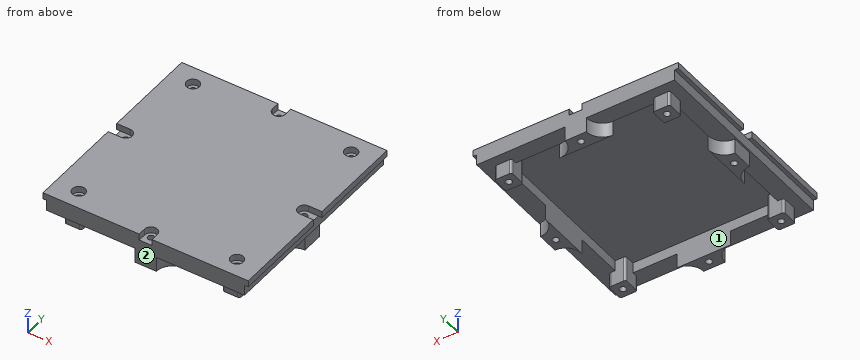
from build123d import *
from build123d.topology import SkipClean

# Parameters (mm, degrees)
SKETCH3_W           = 96
SKETCH3_H           = 3
BOSS_EXTRUDE1_DEPTH = 96
SKETCH4_R           = 1.5
BOSS_EXTRUDE2_DEPTH = 12
SKETCH5_R           = 1.5
BOSS_EXTRUDE3_DEPTH = 12
BOSS_EXTRUDE4_DEPTH = 5
SKETCH10_R          = 1.5
CUT_EXTRUDE1_DEPTH  = 70.519781358
SKETCH11_R          = 3
CUT_EXTRUDE2_DEPTH  = 3
CUT_EXTRUDE3_DEPTH  = 3


with BuildPart() as part:
    # Sketch3 → Boss-Extrude1 (new body)
    with BuildSketch(Plane(origin=(0, 48, 0), x_dir=(1, 0, 0), z_dir=(0, 1, 0))):
        with Locations((0, -1.5)):
            Rectangle(SKETCH3_W, SKETCH3_H)
    extrude(amount=-BOSS_EXTRUDE1_DEPTH)

    # Sketch4 → Boss-Extrude2 (add)
    # profile 1 of 4: a face of its own
    with BuildSketch(Plane(origin=(0, 0, 0), x_dir=(-1, 0, 0), z_dir=(0, 0, -1))):
        with BuildLine():
            Line((38, -12.5), (38, 12.5))
            ThreePointArc((38, 12.5), (40.196699141, 7.196699141), (45.5, 5))
            Line((45.5, 5), (45.5, -5))
            ThreePointArc((45.5, -5), (40.196699141, -7.196699141), (38, -12.5))
        make_face()
        with Locations(Location((41.75, 0, 0), (0, 0, 180))):
            Circle(SKETCH4_R, mode=Mode.SUBTRACT)
    # profile 2 of 4: a face of its own
    with BuildSketch(Plane(origin=(0, 0, 0), x_dir=(-1, 0, 0), z_dir=(0, 0, -1))):
        with BuildLine():
            Line((12.5, 40.5), (-12.5, 40.5))
            ThreePointArc((-12.5, 40.5), (-7.196699141, 42.696699141), (-5, 48))
            Line((-5, 48), (5, 48))
            ThreePointArc((5, 48), (7.196699141, 42.696699141), (12.5, 40.5))
        make_face()
        with Locations(Location((0, 44.25, 0), (0, 0, 180))):
            Circle(SKETCH4_R, mode=Mode.SUBTRACT)
    # profile 3 of 4: a face of its own
    with BuildSketch(Plane(origin=(0, 0, 0), x_dir=(-1, 0, 0), z_dir=(0, 0, -1))):
        with BuildLine():
            Line((-5, -48), (5, -48))
            ThreePointArc((5, -48), (7.196699141, -42.696699141), (12.5, -40.5))
            Line((12.5, -40.5), (-12.5, -40.5))
            ThreePointArc((-12.5, -40.5), (-7.196699141, -42.696699141), (-5, -48))
        make_face()
        with Locations(Location((0, -44.25, 0), (0, 0, 180))):
            Circle(SKETCH4_R, mode=Mode.SUBTRACT)
    # profile 4 of 4: a face of its own
    with BuildSketch(Plane(origin=(0, 0, 0), x_dir=(-1, 0, 0), z_dir=(0, 0, -1))):
        with BuildLine():
            Line((-45.5, 5), (-45.5, -5))
            ThreePointArc((-45.5, -5), (-40.196699141, -7.196699141), (-38, -12.5))
            Line((-38, -12.5), (-38, 12.5))
            ThreePointArc((-38, 12.5), (-40.196699141, 7.196699141), (-45.5, 5))
        make_face()
        with Locations(Location((-41.75, 0, 0), (0, 0, 180))):
            Circle(SKETCH4_R, mode=Mode.SUBTRACT)
    extrude(amount=BOSS_EXTRUDE2_DEPTH)

    # Sketch5 → Boss-Extrude3 (add)
    # profile 1 of 4: a face of its own
    with BuildSketch(Plane(origin=(0, 0, 0), x_dir=(-1, 0, 0), z_dir=(0, 0, -1))):
        with BuildLine():
            Line((-40, 35.5), (-34, 35.5))
            ThreePointArc((-34, 35.5), (-33.292893219, 35.792893219), (-33, 36.5))
            Line((-33, 36.5), (-33, 42.5))
            ThreePointArc((-33, 42.5), (-33.292893219, 43.207106781), (-34, 43.5))
            Line((-34, 43.5), (-40, 43.5))
            ThreePointArc((-40, 43.5), (-40.707106781, 43.207106781), (-41, 42.5))
            Line((-41, 42.5), (-41, 36.5))
            ThreePointArc((-41, 36.5), (-40.707106781, 35.792893219), (-40, 35.5))
        make_face()
        with Locations(Location((-37, 39.5, 0), (0, 0, 90))):
            Circle(SKETCH5_R, mode=Mode.SUBTRACT)
    # profile 2 of 4: a face of its own
    with BuildSketch(Plane(origin=(0, 0, 0), x_dir=(-1, 0, 0), z_dir=(0, 0, -1))):
        with BuildLine():
            Line((33, 36.5), (33, 42.5))
            ThreePointArc((33, 42.5), (33.292893219, 43.207106781), (34, 43.5))
            Line((34, 43.5), (40, 43.5))
            ThreePointArc((40, 43.5), (40.707106781, 43.207106781), (41, 42.5))
            Line((41, 42.5), (41, 36.5))
            ThreePointArc((41, 36.5), (40.707106781, 35.792893219), (40, 35.5))
            Line((40, 35.5), (34, 35.5))
            ThreePointArc((34, 35.5), (33.292893219, 35.792893219), (33, 36.5))
        make_face()
        with Locations(Location((37, 39.5, 0), (0, 0, 90))):
            Circle(SKETCH5_R, mode=Mode.SUBTRACT)
    # profile 3 of 4: a face of its own
    with BuildSketch(Plane(origin=(0, 0, 0), x_dir=(-1, 0, 0), z_dir=(0, 0, -1))):
        with BuildLine():
            Line((-33, -36.5), (-33, -42.5))
            ThreePointArc((-33, -42.5), (-33.292893219, -43.207106781), (-34, -43.5))
            Line((-34, -43.5), (-40, -43.5))
            ThreePointArc((-40, -43.5), (-40.707106781, -43.207106781), (-41, -42.5))
            Line((-41, -42.5), (-41, -36.5))
            ThreePointArc((-41, -36.5), (-40.707106781, -35.792893219), (-40, -35.5))
            Line((-40, -35.5), (-34, -35.5))
            ThreePointArc((-34, -35.5), (-33.292893219, -35.792893219), (-33, -36.5))
        make_face()
        with Locations(Location((-37, -39.5, 0), (0, 0, 90))):
            Circle(SKETCH5_R, mode=Mode.SUBTRACT)
    # profile 4 of 4: a face of its own
    with BuildSketch(Plane(origin=(0, 0, 0), x_dir=(-1, 0, 0), z_dir=(0, 0, -1))):
        with BuildLine():
            Line((40, -35.5), (34, -35.5))
            ThreePointArc((34, -35.5), (33.292893219, -35.792893219), (33, -36.5))
            Line((33, -36.5), (33, -42.5))
            ThreePointArc((33, -42.5), (33.292893219, -43.207106781), (34, -43.5))
            Line((34, -43.5), (40, -43.5))
            ThreePointArc((40, -43.5), (40.707106781, -43.207106781), (41, -42.5))
            Line((41, -42.5), (41, -36.5))
            ThreePointArc((41, -36.5), (40.707106781, -35.792893219), (40, -35.5))
        make_face()
        with Locations(Location((37, -39.5, 0), (0, 0, 90))):
            Circle(SKETCH5_R, mode=Mode.SUBTRACT)
    extrude(amount=BOSS_EXTRUDE3_DEPTH)

    # Sketch8 → Boss-Extrude4 (add)
    with BuildSketch(Plane(origin=(0, 0, 0), x_dir=(-1, 0, 0), z_dir=(0, 0, -1))):
        with BuildLine():
            Line((-38, 40.5), (-12.5, 40.5))
            ThreePointArc((-12.5, 40.5), (-7.196699141, 42.696699141), (-5, 48))
            Line((-5, 48), (-46.25, 48))
            Line((-46.25, 48), (-46.25, -48))
            Line((-46.25, -48), (-5, -48))
            ThreePointArc((-5, -48), (-7.196699141, -42.696699141), (-12.5, -40.5))
            Line((-12.5, -40.5), (-38, -40.5))
            Line((-38, -40.5), (-38, 40.5))
        make_face()
        with BuildLine():
            Line((12.5, 40.5), (38, 40.5))
            Line((38, 40.5), (38, -40.5))
            Line((38, -40.5), (12.5, -40.5))
            ThreePointArc((12.5, -40.5), (7.196699141, -42.696699141), (5, -48))
            Line((5, -48), (46.25, -48))
            Line((46.25, -48), (46.25, 48))
            Line((46.25, 48), (5, 48))
            ThreePointArc((5, 48), (7.196699141, 42.696699141), (12.5, 40.5))
        make_face()
    extrude(amount=BOSS_EXTRUDE4_DEPTH)

    # Sketch10 → Cut-Extrude1 (cut, through all)
    with BuildSketch(Plane.XY.offset(3)):
        with Locations((37, -39.5)):
            Circle(SKETCH10_R)
        with Locations((0, -44.25)):
            Circle(SKETCH10_R)
        with Locations((-37, -39.5)):
            Circle(SKETCH10_R)
        with Locations((-41.75, 0)):
            Circle(SKETCH10_R)
        with Locations((-37, 39.5)):
            Circle(SKETCH10_R)
        with Locations((0, 44.25)):
            Circle(SKETCH10_R)
        with Locations((37, 39.5)):
            Circle(SKETCH10_R)
        with Locations((41.75, 0)):
            Circle(SKETCH10_R)
    extrude(amount=-CUT_EXTRUDE1_DEPTH, mode=Mode.SUBTRACT)

    # Sketch11 → Cut-Extrude2 (cut)
    with SkipClean():  # the faces are left unmerged after this step: merging them gives an invalid solid
        with BuildSketch(Plane.XY.offset(3)):
            with Locations((0, -44.25)):
                Circle(SKETCH11_R)
            with Locations((-37, -39.5)):
                Circle(SKETCH11_R)
            with Locations((-41.75, 0)):
                Circle(SKETCH11_R)
            with Locations((-37, 39.5)):
                Circle(SKETCH11_R)
            with Locations((0, 44.25)):
                Circle(SKETCH11_R)
            with Locations(Location((37, -39.5, 0), (0, 0, 180))):
                Circle(SKETCH11_R)
            with Locations(Location((41.75, 0, 0), (0, 0, 180))):
                Circle(SKETCH11_R)
            with Locations(Location((37, 39.5, 0), (0, 0, 180))):
                Circle(SKETCH11_R)
        extrude(amount=-CUT_EXTRUDE2_DEPTH, mode=Mode.SUBTRACT)

    # Sketch12 → Cut-Extrude3 (cut)
    with BuildSketch(Plane.XY.offset(3)):
        with BuildLine():
            Line((3, -44.25), (3, -51.044271795))
            Line((3, -51.044271795), (-3, -51.044271795))
            Line((-3, -51.044271795), (-3, -44.24999935))
            ThreePointArc((-3, -44.24999935), (-3.25e-07, -47.25), (3, -44.25))
        make_face()
        with BuildLine():
            Line((3, 44.25), (3, 51.044271795))
            Line((3, 51.044271795), (-3, 51.044271795))
            Line((-3, 51.044271795), (-3, 44.24999935))
            ThreePointArc((-3, 44.24999935), (-3.25e-07, 47.25), (3, 44.25))
        make_face()
        with BuildLine():
            Line((41.75, -3), (50.168428877, -3))
            Line((50.168428877, -3), (50.168428877, 3))
            Line((50.168428877, 3), (41.75, 3))
            ThreePointArc((41.75, 3), (44.75, 0), (41.75, -3))
        make_face()
        with BuildLine():
            Line((-50.168428877, -3), (-50.168428877, 3))
            Line((-50.168428877, 3), (-41.75, 3))
            ThreePointArc((-41.75, 3), (-44.75, 0), (-41.75, -3))
            Line((-41.75, -3), (-50.168428877, -3))
        make_face()
    extrude(amount=-CUT_EXTRUDE3_DEPTH, mode=Mode.SUBTRACT)


solid = part.part
Geometry check sheet. Reference: the model listing, model coordinates, mm. Face numbers are marked on the shaded views. A direction names the side the tool comes from. Give positions to 0.01 mm unless a question says otherwise; leave off trailing zeros. Loops run counter-clockwise (first coordinate to the right, second up) from the corner with the lowest first, then second, coordinate; pieces in that order, holes last. Notation, with made-up numbers: M 47,83 L 103,83 A31 cw 103,117 Z; hole C 16,-7.5 d11. An arc over 180 degrees is marked long. Answer as a JSON object with one key per item and string values. Group by question number.
Item 1: Sectioned sample at C-C on y = 27. Record the boundary of the cut face in (x, z).
Item 2: Material ranges on L1, parallel to Y at x = 37, z = -2.25; L2, parallel to Y at x = -37, z = 0.5; L3, parallel to X at y = -37.5, z = -8, recorded low to high.
Item 3: Sectioned sample at A-A on z = -3.5. Give the number of separate pieces and of enclosed holes in the cut face, plus the area to 3 significant figures.
Item 4: Access from +Z, -Z, +X, -X, +Y, -Y to the whole of each face (thin tool, end or side, straight path). Record for the marked faces 1 and 2.
Item 5: Gauge pin test, flat ends, axial feed: pin 1 (6 mm diameter, centred on x = 28, y = 8, fed in from -Z); pin 2 (6.5 mm diameter, centred on x = 37.5, y = 39, fed in from +Z); pin 3 (2.5 mm diameter, centred on x = 41.75, y = 0, fed in from +Z); pin 4 (3 mm diameter, centred on y = 37, z = -7.5, fed in from -X). Record the tip position at first contact, or that the pin passes through.
Item 6: Sectioned sample at B-B on x = -23.5. Record the boundary of the cut face in (y, z).
Findings below:
{
 "1": {"outline": "M -48,0 L -46.25,0 L -46.25,-5 L -38,-5 L -38,0 L 38,0 L 38,-5 L 46.25,-5 L 46.25,0 L 48,0 L 48,3 L -48,3 Z"},
 "2": {"L1": "-48 to -41, -38 to -35.5, 35.5 to 38, 41 to 48", "L2": "-48 to -42.5, -36.5 to 36.5, 42.5 to 48", "L3": "-41 to -33, 33 to 41"},
 "3": {"separate pieces": "1", "enclosed holes": "9", "area": "2,770 mm2"},
 "4": {"face 1": "-Z", "face 2": "+Z, -Z, +X, -X, -Y"},
 "5": {"pin 1": "z = 0", "pin 2": "z = 3", "pin 3": "through", "pin 4": "x = -41"},
 "6": {"outline": "M -48,-5 L -40.5,-5 L -40.5,0 L 40.5,0 L 40.5,-5 L 48,-5 L 48,3 L -48,3 Z"}
}
